```python
from build123d import *
from build123d.topology import SkipClean

# Parameters (mm, degrees)
SKETCH1_R           = 17.5
SKETCH1_R_2         = 16.3
BOSS_EXTRUDE1_DEPTH = 10
BOSS_EXTRUDE2_START = 6
SKETCH2_R           = 17.5
SKETCH2_R_2         = 8
BOSS_EXTRUDE2_DEPTH = 6
BOSS_EXTRUDE3_DEPTH = 6
FILLET1_R           = 10


with BuildPart() as part:
    # Sketch1 → Boss-Extrude1 (new body)
    with BuildSketch(Plane(origin=(0, 0, 0), x_dir=(1, 0, 0), z_dir=(0, 1, 0))):
        with Locations(Location((0, 0, 0), (0, 0, 270))):
            Circle(SKETCH1_R)
        with Locations(Location((0, 0, 0), (0, 0, 270))):
            Circle(SKETCH1_R_2, mode=Mode.SUBTRACT)
    extrude(amount=BOSS_EXTRUDE1_DEPTH)

    # Sketch2 → Boss-Extrude2 (add)
    with BuildSketch(Plane.XZ.offset(BOSS_EXTRUDE2_START)):
        with Locations(Location((0, 0, 0), (0, 0, 270))):
            Circle(SKETCH2_R)
        with Locations(Location((0, 0, 0), (0, 0, 270))):
            Circle(SKETCH2_R_2, mode=Mode.SUBTRACT)
    extrude(amount=-BOSS_EXTRUDE2_DEPTH)

    # Sketch4 → Boss-Extrude3 (add)
    with SkipClean():  # the faces are left unmerged after this step: merging them gives an invalid solid
        with BuildSketch(Plane.XZ.offset(6)):
            with BuildLine():
                Line((-28.394541729, 8), (-8, 8))
                Line((-8, 8), (-8, -8))
                Line((-8, -8), (-28.394541729, -8))
                ThreePointArc((-28.394541729, -8), (-29.5, 0), (-28.394541729, 8))
            make_face()
            with BuildLine():
                Line((28.394541729, -8), (8, -8))
                Line((8, -8), (8, 8))
                Line((8, 8), (28.394541729, 8))
                ThreePointArc((28.394541729, 8), (29.5, 0), (28.394541729, -8))
            make_face()
        extrude(amount=-BOSS_EXTRUDE3_DEPTH)

    # Fillet1
    # the kernel refuses this fillet: 10 mm, written as the material it adds along each edge
    with BuildSketch(Plane(origin=(-15.564382416, 0, 8), x_dir=(0.5598300249695263, 0, 0.8286074722947046), z_dir=(0, -1, 0)), Plane(origin=(15.564382416, 0, -8), x_dir=(-0.5598300249695256, 0, -0.828607472294705), z_dir=(0, -1, 0))) as fillet1_piece_1:
        with BuildLine():
            CenterArc((5.36026839, 9.928802155), FILLET1_R, 214.044043652, 49.114807107)
            Line((-2.925806333, 4.330501905), (0, 0))
            ThreePointArc((0, 0), (2.084548818, 0.124596228), (4.169097637, 0))
        make_face()
    extrude(amount=6)
    with BuildSketch(Plane(origin=(-15.564382416, 0, -8), x_dir=(0.5598300249695259, 0, -0.8286074722947048), z_dir=(0, -1, 0)), Plane(origin=(15.564382416, 0, 8), x_dir=(-0.5598300249695263, 0, 0.8286074722947046), z_dir=(0, -1, 0))) as fillet1_piece_2:
        with BuildLine():
            CenterArc((5.36026839, -9.928802155), FILLET1_R, 96.84114924, 49.114807107)
            Line((-2.925806333, -4.330501905), (0, 0))
            ThreePointArc((0, 0), (2.084548818, -0.124596228), (4.169097637, 0))
        make_face()
    extrude(amount=6)


solid = part.part
```
The model under review builds one solid part; all positions refer to its coordinate system, in mm. A direction names the side the tool comes from. Coordinates: 2 decimals unless noted, no trailing zeros. Write each loop counter-clockwise with the first axis right and the second up, starting at its lowest first coordinate (ties: lowest second). Pieces come first, ordered by that corner, then holes.
1) We need section D-D on y = 7. State the section outline as (x, z) points.
2) We need section B-B on z = -3. State the section outline as (x, y) points, then the cut area to 3 significant figures.
3) To check wall thickness, follow probe 1 along Z at (x, y) = (0, 4.5); probe 2 along Z at (x, y) = (-8, 7.25). State the ranges of each line that lie inside material, in increasing order.
4) We need section C-C on z = 9. State the section outline as (x, y) points, then the cut area to 3 significant figures.
5) Clearance check with flat-ended pins moving along their axes: pin 1 Ø3 at (x, y) = (23.5, -2.5) entering from -Z; pin 2 Ø3 at (x, z) = (-19, -9.5) entering from +Y; pin 3 Ø6 at (x, y) = (-20.5, -2.5) entering from -Z. State where each tip first meets the part, or that it passes through.
6) We need section A-A on y = -3. State the section outline as (x, z) points.
7) Machinability: for faces 1 (the face through (-25, -3, -8)), 2 (the face through (25, -3, -8)), 3 (the face through (-25, -3, 8)), 4 (the face through (-9.918, 4.93, -12.935)), which of the approach directions +Z, -Z, +X, -X, +Y, -Y give a long, thin tool a straight path to every point of the face, cutting with its end or side? Answer none if there is none.
Answer list:
1. outline: circle Ø35 at (0, 0); hole circle Ø32.6 at (0, 0)
2. outline: (-29.35, -6) - (-7.42, -6) - (-7.42, 0) - (-16.02, 0) - (-16.02, 10) - (-17.24, 10) - (-17.24, 0) - (-29.35, 0) - close; (7.42, -6) - (29.35, -6) - (29.35, 0) - (17.24, 0) - (17.24, 10) - (16.02, 10) - (16.02, 0) - (7.42, 0) - close
2. area: 288 mm2
3. probe 1: z = -17.5 to -16.3, 16.3 to 17.5
3. probe 2: z = -15.56 to -14.2, 14.2 to 15.56
4. outline: (-16.43, -6) - (16.43, -6) - (16.43, 0) - (15.01, 0) - (15.01, 10) - (13.59, 10) - (13.59, 0) - (-13.59, 0) - (-13.59, 10) - (-15.01, 10) - (-15.01, 0) - (-16.43, 0) - close
4. area: 226 mm2
5. pin 1: stops at z = -8
5. pin 2: stops at y = 0
5. pin 3: stops at z = -8.56
6. outline: (-28.39, -8) - (-20.79, -8) arc R10 cw to (-13.23, -11.45) arc R17.5 ccw to (13.23, -11.45) arc R10 cw to (20.79, -8) - (28.39, -8) arc R29.5 ccw to (28.39, 8) - (20.79, 8) arc R10 cw to (13.23, 11.45) arc R17.5 ccw to (-13.23, 11.45) arc R10 cw to (-20.79, 8) - (-28.39, 8) arc R29.5 ccw to start; hole circle Ø16 at (0, 0)
7. face 1: -Z, -X, +Y, -Y
7. face 2: -Z, +X, +Y, -Y
7. face 3: +Z, -X, +Y, -Y
7. face 4: +Y
